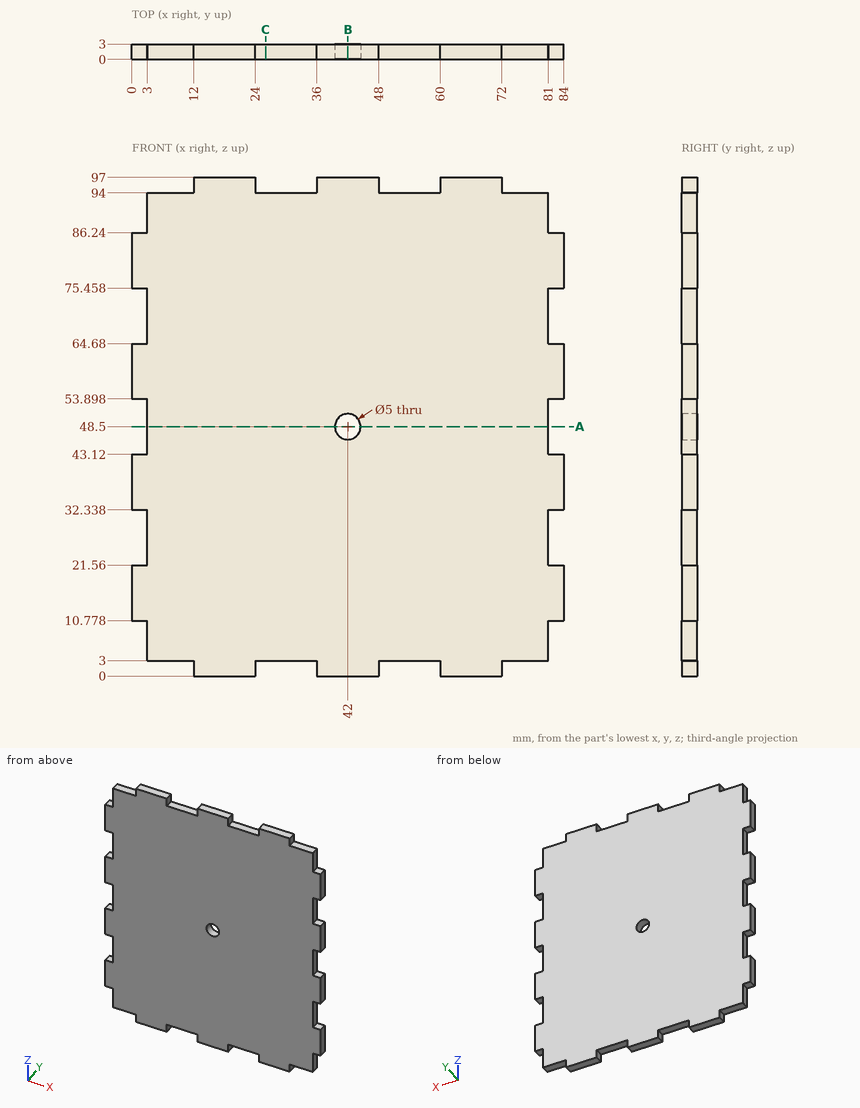
For this review, use the dimensioned drawing (mm, ordinates from the lowest corner) and the shaded views. Give positions to 0.01 mm unless a question says otherwise; leave off trailing zeros. Loops run counter-clockwise (first coordinate to the right, second up) from the corner with the lowest first, then second, coordinate; pieces in that order, holes last.
Item 1: Take a section at A-A, the plane z = 48.5. State the section outline as (x, y) points, and give its area (3 significant figures).
Item 2: Insertion check: pin 1 (1.5 mm diameter, centred on y = 1, z = 6.5, fed in from -X); pin 2 (1.5 mm diameter, centred on x = 82, y = 2, fed in from -Z); pin 3 (0.9 mm diameter, centred on x = 82.5, y = 1, fed in from +Z). Each pin has a flat end and moves straight along its axis. Give the tip position at first contact, or say it passes through.
Item 3: Take a section at C-C, the plane x = 26. State the section outline as (y, z) points.
Item 4: Take a section at B-B, the plane x = 42. State the section outline as (y, z) points.
Item 5: For line 1 along X through (y, z) = (1.05, 48.5); line 2 along Z through (x, y) = (26, 2.6); line 3 along X through (y, z) = (1.45, 4.5), list the stretches that pass through material, from the lowest coordinate up.
Calculated:
1. outline: (3, 0) - (39.5, 0) - (39.5, 3) - (3, 3) - close; (44.5, 0) - (81, 0) - (81, 3) - (44.5, 3) - close
1. area: 219 mm2
2. pin 1: stops at x = 3
2. pin 2: stops at z = 10.78
2. pin 3: stops at z = 86.24
3. outline: (0, 3) - (3, 3) - (3, 94) - (0, 94) - close
4. outline: (0, 0) - (3, 0) - (3, 46) - (0, 46) - close; (0, 51) - (3, 51) - (3, 97) - (0, 97) - close
5. line 1: x = 3 to 39.5, 44.5 to 81
5. line 2: z = 3 to 94
5. line 3: x = 3 to 81
